Read the model definition and answer for the solid it produces. Units are mm, in the model's axes. Give positions to 0.01 mm unless a question says otherwise; leave off trailing zeros. Order: outer loops, then holes, each group sorted by start corner. A loop starts at its lowest first (then second) coordinate and runs counter-clockwise, first axis right, second up.
```python
from build123d import *

# Parameters (mm, degrees)
BOSS_EXTRUDE2_DEPTH = 127
SKETCH3_R           = 57.15
CUT_EXTRUDE1_DEPTH  = 62
CUT_EXTRUDE2_DEPTH  = 128


with BuildPart() as part:
    # Sketch2 → Boss-Extrude2 (new body)
    with BuildSketch(Plane.XY):
        Polygon((0, 0), (0, -127), (63.5, -127), (127, 0), align=None)
    extrude(amount=BOSS_EXTRUDE2_DEPTH)

    # Sketch3 → Cut-Extrude1 (cut)
    with BuildSketch(Plane.ZY):
        with Locations((63.5, -63.5)):
            Circle(SKETCH3_R)
    extrude(amount=-CUT_EXTRUDE1_DEPTH, mode=Mode.SUBTRACT)

    # Sketch4 → Cut-Extrude2 (cut, through all)
    with BuildSketch(Plane.ZY):
        with BuildLine():
            Line((127, 0), (63.5, 0))
            ThreePointArc((63.5, 0), (108.401280605, -18.598719395), (127, -63.5))
            Line((127, -63.5), (127, 0))
        make_face()
        with BuildLine():
            Line((63.5, 0), (0, 0))
            Line((0, 0), (0, -63.5))
            ThreePointArc((0, -63.5), (18.598719395, -18.598719395), (63.5, 0))
        make_face()
        with BuildLine():
            ThreePointArc((63.5, -127), (18.598719395, -108.401280605), (0, -63.5))
            Line((0, -63.5), (0, -127))
            Line((0, -127), (63.5, -127))
        make_face()
        with BuildLine():
            Line((127, -127), (127, -63.5))
            ThreePointArc((127, -63.5), (108.401280605, -108.401280605), (63.5, -127))
            Line((63.5, -127), (127, -127))
        make_face()
    extrude(amount=-CUT_EXTRUDE2_DEPTH, mode=Mode.SUBTRACT)


solid = part.part
```
1) For a pull along Y with two mould halves and no side action, classify faces 1 (the face through (0, -11, 40)), 2 (the face through (95, -64, 63)), 3 (the face through (30.6, -46.3, 118)) as released by +Y, released by -Y, zero draft, split by the parting line, or undercut.
Final values:
face 1: zero draft
face 2: released by -Y
face 3: undercut
2) The part is cut by section A-A on x = 12.5. Determine the outline of the cut face in (y, z).
Final values:
outline: circle Ø127 at (-63.5, 63.5); hole circle Ø114.3 at (-63.5, 63.5)
3) Given pin 1 (5 mm diameter, centred on y = -40.5, z = 99, fed in from -X); pin 2 (8 mm diameter, centred on x = 76.5, z = 113, fed in from -Y); pin 3 (1.5 mm diameter, centred on y = -42.5, z = 55.5, fed in from +X) (3 decimals), each flat-ended and moving along its own axis, determine where each tip first touches the part or whether it passes through.
Final values:
pin 1: stops at x = 62
pin 2: stops at y = -106.59
pin 3: stops at x = 106.125
4) The part is cut by section C-C on y = -53.5. Determine the outline of the cut face in (x, z).
Final values:
outline: (0, 0.79) - (100.25, 0.79) - (100.25, 126.21) - (0, 126.21) - (0, 119.77) - (62, 119.77) - (62, 7.23) - (0, 7.23) - close
5) The part is cut by section B-B on z = 39.5. Determine the outline of the cut face in (x, y), and give its area (3 significant figures).
Final values:
outline: (0, -122.29) - (65.86, -122.29) - (124.64, -4.71) - (0, -4.71) - (0, -11.63) - (62, -11.63) - (62, -115.37) - (0, -115.37) - close
area: 4,770 mm2
6) Consider L1, parallel to Z at x = 35, y = -63; L2, parallel to Y at x = 40, z = 63.5; L3, parallel to Z at x = 7, y = -12. Determine where each line is inside the solid, lowest interval first.
Final values:
L1: z = 0 to 6.35, 120.65 to 127
L2: y = -127 to -120.65, -6.35 to 0
L3: z = 26.35 to 38.72, 88.28 to 100.65
7) The part is cut by section D-D on x = 88. Determine the outline of the cut face in (y, z).
Final values:
outline: (-78, 1.68) arc R63.5 ccw (long way) to (-78, 125.32) - close
